from build123d import *

# Parameters (mm, degrees)
F2_R     = 5.25
F3_DEPTH = 20
F4_DEPTH = 2
F5_DEPTH = 18
F6_SIZE  = 0.6


with BuildPart() as f3:
    # F2 (on Top) → F3 (new body)
    with BuildSketch(Plane.XY):
        Polygon((5.25, 40.25), (0, 40.25), (0, 20), (0, 16.3397459622), (0, 3.6602540378), (0, 0), (20, 0), (20, 40.25), (14.75, 40.25), align=None)
        with Locations((10, 10.25)):
            Circle(F2_R, mode=Mode.SUBTRACT)
        Polygon((0, 16.3397459622), (0, 20), (-5, 20), (-5, 15), align=None)
        Polygon((0, 0), (0, 3.6602540378), (-5, 5), (-5, 0), align=None)
    extrude(amount=F3_DEPTH)

    # F2 (on Top) → F4 (join)
    with BuildSketch(Plane.XY):
        Polygon((0, 3.6602540378), (0, 16.3397459622), (-5, 15), (-5, 5), align=None)
    extrude(amount=F4_DEPTH)

    # F2 (on Top) → F5 (join)
    with BuildSketch(Plane.XY):
        Polygon((4.0442286341, 44.75), (5.25, 40.25), (14.75, 40.25), (15.9557713659, 44.75), align=None)
    extrude(amount=F5_DEPTH)

    # F6
    f6_edges = [f3.edges().sort_by_distance(p)[0] for p in [
        (0, 30.125, 0),
        (-2.5, 20, 0),
        (-5, 10, 0),
        (7.5, 0, 0),
        (20, 20.125, 0),
        (17.375, 40.25, 0),
        (15.352886, 42.5, 0),
        (10, 44.75, 0),
        (4.647114, 42.5, 0),
        (2.625, 40.25, 0),
        (4.75, 10.25, 0),
        (0, 30.125, 20),
        (-2.5, 20, 20),
        (-5, 17.5, 20),
        (-2.5, 15.669873, 20),
        (0, 10, 20),
        (-2.5, 4.330127, 20),
        (-5, 2.5, 20),
        (7.5, 0, 20),
        (20, 20.125, 20),
        (10, 40.25, 20),
        (4.75, 10.25, 20),
        (-5, 0, 10),
        (20, 0, 10),
        (20, 40.25, 10),
        (0, 20, 10),
        (-5, 20, 10),
        (0, 40.25, 10),
    ]]
    chamfer(f6_edges, length=F6_SIZE)


solid = f3.part
Input: part model. Units: mm. Frame: model coordinates. A direction names the side the tool comes from. Coordinates: 2 decimals unless noted, no trailing zeros. Order: outer loops, then holes, each group sorted by start corner. A loop starts at its lowest first (then second) coordinate and runs counter-clockwise, first axis right, second up.
1. Access query for faces 4 (the flat face through (0, 10, 11)), 5 (the flat face through (5.024, 42.236, 0.304)), 6 (the flat face through (4.64, 42.53, 9.18)). Directions: +Z, -Z, +X, -X, +Y, -Y. A direction counts if a zero-diameter tool reaches every point of the face in a straight line with its end or side. Return the directions, or none.
Checked values:
face 4: +Z
face 5: -Z, -X
face 6: +Z, -Z, -X
2. Cut plane D-D, the plane y = 29. Return loops of the section in (x, z), plus the area to 3 significant figures.
Checked values:
outline: (0, 0.6) - (0.6, 0) - (19.4, 0) - (20, 0.6) - (20, 19.4) - (19.4, 20) - (0.6, 20) - (0, 19.4) - close
area: 399 mm2
3. Cut plane B-B, the plane y = 10.25. Return loops of the section in (x, z).
Checked values:
outline: (-5, 0.6) - (-4.4, 0) - (4.15, 0) - (4.75, 0.6) - (4.75, 19.4) - (4.15, 20) - (0.6, 20) - (0, 19.4) - (0, 2) - (-5, 2) - close; (15.25, 0.6) - (15.85, 0) - (19.4, 0) - (20, 0.6) - (20, 19.4) - (19.4, 20) - (15.85, 20) - (15.25, 19.4) - close
4. Contact query for flat-ended pins moving along their axis: P1, Ø8, axis at y = 19.5, z = 10.5, coming from the -X side; P2, Ø1.9, axis at x = -2.5, z = 6, coming from the +Y side; P3, Ø8, axis at y = 10, z = 12.5, coming from the -X side; P4, Ø5.5, axis at x = -3.5, y = 7.5, coming from the +Z side. Output: stop coordinate, or through.
Checked values:
P1: stops at x = -5
P2: stops at y = 20
P3: stops at x = 0
P4: stops at z = 2
5. Cut plane C-C, the plane z = 3.25. Return loops of the section in (x, y).
Checked values:
outline: (-5, 0.6) - (-4.4, 0) - (19.4, 0) - (20, 0.6) - (20, 39.65) - (19.4, 40.25) - (14.75, 40.25) - (15.96, 44.75) - (4.04, 44.75) - (5.25, 40.25) - (0.6, 40.25) - (0, 39.65) - (0, 20.6) - (-0.6, 20) - (-4.4, 20) - (-5, 19.4) - (-5, 15) - (0, 16.34) - (0, 3.66) - (-5, 5) - close; hole circle Ø10.5 at (10, 10.25)
6. Draft query along Y for faces 1 (the cylindrical face through (12.82, 14.68, 9.87)), 2 (the flat face through (10, 43, 18)), 3 (the flat face through (-2, 20, 10)). Return one class per face: +Y half, -Y half, draft (parallel to the pull), parting line (faces both ways), or undercut.
Checked values:
face 1: undercut
face 2: draft
face 3: +Y half
7. Ray query, line 1 along Y through (x, z) = (10, 14.5); line 2 along X through (y, z) = (8, 8); line 3 along Z through (x, y) = (-3, 14). Return the intervals inside material, ascending.
Checked values:
line 1: y = 0 to 5, 15.5 to 44.75
line 2: x = 0 to 5.26, 14.74 to 20
line 3: z = 0 to 2
8. Cut plane A-A, the plane x = 10. Return loops of the section in (y, z).
Checked values:
outline: (0, 0.6) - (0.6, 0) - (4.4, 0) - (5, 0.6) - (5, 19.4) - (4.4, 20) - (0.6, 20) - (0, 19.4) - close; (15.5, 0.6) - (16.1, 0) - (44.15, 0) - (44.75, 0.6) - (44.75, 18) - (40.25, 18) - (40.25, 19.4) - (39.65, 20) - (16.1, 20) - (15.5, 19.4) - close
